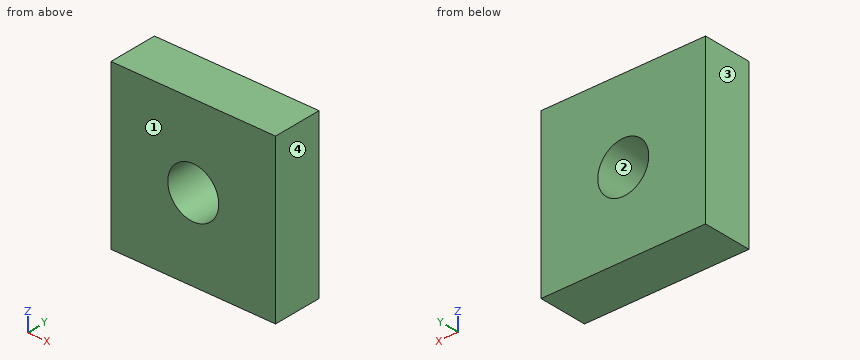
```python
from build123d import *

# Parameters (mm, degrees)
CROQUIS1_W              = 10
CROQUIS1_H              = 10
CROQUIS1_R              = 1.55
SALIENTE_EXTRUIR1_DEPTH = 3


with BuildPart() as part:
    # Croquis1 → Saliente-Extruir1 (new body)
    with BuildSketch(Plane(origin=(0, 0, 0), x_dir=(1, 0, 0), z_dir=(0, 1, 0))):
        Rectangle(CROQUIS1_W, CROQUIS1_H)
        with Locations(Location((0, 0, 0), (0, 0, 270))):
            Circle(CROQUIS1_R, mode=Mode.SUBTRACT)
    extrude(amount=SALIENTE_EXTRUIR1_DEPTH)


solid = part.part
```
Part model, mm, in its own coordinate system. Face numbers are marked on the shaded views. Round coordinates to 2 decimals unless told otherwise and drop trailing zeros. Order: outer loops, then holes, each group sorted by start corner. A loop starts at its lowest first (then second) coordinate and runs counter-clockwise, first axis right, second up. Notation, with made-up numbers: M 78.25,-15 L 94.25,-15 A7 cw 94.25,-7 Z; hole C 32.5,2.5 d11. An arc over 180 degrees is marked long. Put each result on its own line as item: value. Start each with the question number.
1. Drill centre lines: probe 1 along X at (y, z) = (2, 0); probe 2 along Z at (x, y) = (1, 1.4). Where is each one in solid material? Low to high. Write a range as [from, to].
2. Slice it at C-C on y = 2.45. List the corners of the cut face in (x, z).
3. Slice it at B-B on x = 0. List the corners of the cut face in (y, z).
4. Two-plate mould, pull along X, no slides. Class the marked faces 1, 2, 3 and 4: +X half, -X half, draft (parallel to the pull), parting line (faces both ways), or undercut.
5. Slice it at A-A on z = 0. List the corners of the cut face in (x, y), then the cut area to 3 significant figures.
Findings:
1. probe 1: [-5, -1.55], [1.55, 5]
1. probe 2: [-5, -1.18], [1.18, 5]
2. outline: M -5,-5 L 5,-5 L 5,5 L -5,5 Z; hole C 0,0 d3.1
3. outline: M 0,-5 L 3,-5 L 3,-1.55 L 0,-1.55 Z; M 0,1.55 L 3,1.55 L 3,5 L 0,5 Z
4. face 1: draft
4. face 2: undercut
4. face 3: -X half
4. face 4: +X half
5. outline: M -5,0 L -1.55,0 L -1.55,3 L -5,3 Z; M 1.55,0 L 5,0 L 5,3 L 1.55,3 Z
5. area: 20.7 mm2
